Read the model definition and answer for the solid it produces. Units are mm, in the model's axes. A direction names the side the tool comes from. Coordinates: 2 decimals unless noted, no trailing zeros. Loops run counter-clockwise (first coordinate to the right, second up) from the corner with the lowest first, then second, coordinate; pieces in that order, holes last. Notation, with made-up numbers: (26.5, 7.25) -> (82.5, 7.25) arc R8 ccw to (82.5, 15.25) -> close; hole circle Ø11 at (76.25, 0). An arc over 180 degrees is marked (long way). One line per question, with ' | ' between items. Start each with the question number.
```python
from build123d import *

# Parameters (mm, degrees)
SKETCH1_W           = 200
SKETCH1_H           = 42
BOSS_EXTRUDE1_DEPTH = 6.35
SKETCH4_R           = 2.286
CUT_EXTRUDE3_DEPTH  = 7.35
CHAMFER1_SIZE       = 5
SKETCH9_R           = 2.286
CUT_EXTRUDE8_DEPTH  = 7.35
SKETCH12_R          = 2.286
CUT_EXTRUDE11_DEPTH = 7.35
SKETCH13_R          = 2.286
CUT_EXTRUDE12_DEPTH = 10


with BuildPart() as part:
    # Sketch1 → Boss-Extrude1 (new body)
    with BuildSketch(Plane.XY):
        Rectangle(SKETCH1_W, SKETCH1_H)
    extrude(amount=BOSS_EXTRUDE1_DEPTH)

    # Sketch4 → Cut-Extrude3 (cut, through all)
    with BuildSketch(Plane.XY.offset(6.35)):
        with Locations((-76, 0)):
            Circle(SKETCH4_R)
    extrude(amount=-CUT_EXTRUDE3_DEPTH, mode=Mode.SUBTRACT)

    # Chamfer1
    chamfer1_edges = [part.edges().sort_by_distance(p)[0] for p in [
        (100, -21, 3.175),
        (-100, -21, 3.175),
        (-100, 21, 3.175),
        (100, 21, 3.175),
    ]]
    chamfer(chamfer1_edges, length=CHAMFER1_SIZE)

    # Sketch9 → Cut-Extrude8 (cut, through all)
    with BuildSketch(Plane.XY.offset(6.35)):
        with Locations((80, 0)):
            Circle(SKETCH9_R)
    extrude(amount=-CUT_EXTRUDE8_DEPTH, mode=Mode.SUBTRACT)

    # Sketch12 → Cut-Extrude11 (cut, through all)
    with BuildSketch(Plane.XY.offset(6.35)):
        with Locations((-93, 0)):
            Circle(SKETCH12_R)
    extrude(amount=-CUT_EXTRUDE11_DEPTH, mode=Mode.SUBTRACT)

    # Sketch13 → Cut-Extrude12 (cut)
    with BuildSketch(Plane.XY.offset(6.35)):
        Polygon((45, 21), (50, 16), (50, -16), (45, -21), (95, -21), (100, -16), (100, 16), (95, 21), align=None)
        with Locations((80, 0)):
            Circle(SKETCH13_R, mode=Mode.SUBTRACT)
        with BuildLine():
            ThreePointArc((35, -7.46), (37.54, -10), (35, -12.54))
            Line((35, -12.54), (-25, -12.54))
            ThreePointArc((-25, -12.54), (-27.54, -10), (-25, -7.46))
            Line((-25, -7.46), (35, -7.46))
        make_face()
        with BuildLine():
            Line((-25, 7.46), (35, 7.46))
            ThreePointArc((35, 7.46), (37.54, 10), (35, 12.54))
            Line((35, 12.54), (-25, 12.54))
            ThreePointArc((-25, 12.54), (-27.54, 10), (-25, 7.46))
        make_face()
    extrude(amount=-CUT_EXTRUDE12_DEPTH, mode=Mode.SUBTRACT)


solid = part.part
```
(1) Section A-A on y = -10 is taken. Write down the section's boundary in (x, z), plus the area to 3 significant figures.
(2) Section C-C on x = -20.5 is taken. Write down the section's boundary in (y, z), plus the area to 3 significant figures.
(3) Section B-B on y = 0 is taken. Write down the section's boundary in (x, z), plus the area to 3 significant figures.
(4) This flat-tipped pin is pushed along its axis until it touches: pin 1 Ø4 at (x, y) = (-93, 0) entering from +Z. Where does it stop, or does it pass through?
(5) Section D-D on z = 5 is taken. Write down the section's boundary in (x, y).
(6) Find the intervals of material crossed by probe 1 along Y at (x, z) = (18, 0.5); probe 2 along Y at (x, z) = (-93, 4.5); probe 3 along X at (y, z) = (-9, 1), in increasing order. Write a range as from..to.
(7) Determine the mould class of faces 1 (the flat face through (-97, 19, 3)), 2 (the cylindrical face through (-77.685, 1.545, 3.219)), 3 (the flat face through (-26, 21, 3)) for opening direction X: +X half, -X half, draft (parallel to the pull), parting line (faces both ways), or undercut.
(8) A tool of negligible diameter and unlimited length cuts with its end or side. For faces 4 (the flat face through (5, 7.46, 3)), 5 (the flat face through (-100, 0, 3)), from which of +Z, -Z, +X, -X, +Y, -Y can it reach the whole face along a straight path? Write none if from no direction.
Working result:
1) outline: (-100, 0) -> (-27.54, 0) -> (-27.54, 6.35) -> (-100, 6.35) -> close; (37.54, 0) -> (50, 0) -> (50, 6.35) -> (37.54, 6.35) -> close | area: 539 mm2
2) outline: (-21, 0) -> (-12.54, 0) -> (-12.54, 6.35) -> (-21, 6.35) -> close; (-7.46, 0) -> (7.46, 0) -> (7.46, 6.35) -> (-7.46, 6.35) -> close; (12.54, 0) -> (21, 0) -> (21, 6.35) -> (12.54, 6.35) -> close | area: 202 mm2
3) outline: (-100, 0) -> (-95.29, 0) -> (-95.29, 6.35) -> (-100, 6.35) -> close; (-90.71, 0) -> (-78.29, 0) -> (-78.29, 6.35) -> (-90.71, 6.35) -> close; (-73.71, 0) -> (50, 0) -> (50, 6.35) -> (-73.71, 6.35) -> close | area: 894 mm2
4) pin 1: passes through
5) outline: (-100, -16) -> (-95, -21) -> (45, -21) -> (50, -16) -> (50, 16) -> (45, 21) -> (-95, 21) -> (-100, 16) -> close; hole circle Ø4.57 at (-93, 0); hole circle Ø4.57 at (-76, 0); hole (-25, -12.54) -> (35, -12.54) arc R2.54 ccw to (35, -7.46) -> (-25, -7.46) arc R2.54 ccw to start; hole (-25, 7.46) -> (35, 7.46) arc R2.54 ccw to (35, 12.54) -> (-25, 12.54) arc R2.54 ccw to start
6) probe 1: y = -21..-12.54, -7.46..7.46, 12.54..21 | probe 2: y = -21..-2.29, 2.29..21 | probe 3: x = -100..-27.33, 37.33..50
7) face 1: -X half | face 2: undercut | face 3: draft
8) face 4: +Z, -Z | face 5: +Z, -Z, -X, +Y, -Y
